```python
from build123d import *

# Parameters (mm, degrees)
CROQUIS1_R                 = 15
SALIENTE_EXTRUIR1_DEPTH    = 22
CROQUIS2_R                 = 10.5
CORTAR_EXTRUIR1_DEPTH      = 16
CORTAR_EXTRUIR2_START      = -1
CORTAR_EXTRUIR2_DEPTH      = 1
CORTAR_EXTRUIR3_START      = -1
CROQUIS5_R                 = 11
CROQUIS5_R_2               = 10.5
CORTAR_EXTRUIR3_DEPTH      = 1
CORTAR_EXTRUIR4_DEPTH      = 31.56141358
CORTAR_EXTRUIR4_DEPTH_BACK = 31.56141358
CROQUIS6_R                 = 1.25


with BuildPart() as part:
    # Croquis1 → Saliente-Extruir1 (new body)
    with BuildSketch(Plane.XY):
        Circle(CROQUIS1_R)
    extrude(amount=SALIENTE_EXTRUIR1_DEPTH)

    # Croquis2 → Cortar-Extruir1 (cut)
    with BuildSketch(Plane.XY.offset(22)):
        Circle(CROQUIS2_R)
    extrude(amount=-CORTAR_EXTRUIR1_DEPTH, mode=Mode.SUBTRACT)

    # Croquis3 → Cortar-Extruir2 (cut)
    with BuildSketch(Plane(origin=(0, 0, 0), x_dir=(-1, 0, 0), z_dir=(0, 0, -1)).offset(CORTAR_EXTRUIR2_START)):
        with BuildLine():
            ThreePointArc((1.25, 10.425329731), (0, 10.5), (-1.25, 10.425329731))
            Line((-1.25, 10.425329731), (-1.25, 9.5))
            Line((-1.25, 9.5), (1.25, 9.5))
            Line((1.25, 9.5), (1.25, 10.425329731))
        make_face()
        with BuildLine():
            Line((-7.602241336, 5.832531755), (-8.40360039, 6.29519662))
            ThreePointArc((-8.40360039, 6.29519662), (-9.09326674, 5.25), (-9.65360039, 4.130133111))
            Line((-9.65360039, 4.130133111), (-8.852241336, 3.667468245))
            Line((-8.852241336, 3.667468245), (-7.602241336, 5.832531755))
        make_face()
        with BuildLine():
            ThreePointArc((9.65360039, 4.130133111), (9.09326674, 5.25), (8.40360039, 6.29519662))
            Line((8.40360039, 6.29519662), (7.602241336, 5.832531755))
            Line((7.602241336, 5.832531755), (8.852241336, 3.667468245))
            Line((8.852241336, 3.667468245), (9.65360039, 4.130133111))
        make_face()
        with BuildLine():
            ThreePointArc((8.40360039, -6.29519662), (9.09326674, -5.25), (9.65360039, -4.130133111))
            Line((9.65360039, -4.130133111), (8.852241336, -3.667468245))
            Line((8.852241336, -3.667468245), (7.602241336, -5.832531755))
            Line((7.602241336, -5.832531755), (8.40360039, -6.29519662))
        make_face()
        with BuildLine():
            Line((-1.25, -9.5), (-1.25, -10.425329731))
            ThreePointArc((-1.25, -10.425329731), (0, -10.5), (1.25, -10.425329731))
            Line((1.25, -10.425329731), (1.25, -9.5))
            Line((1.25, -9.5), (-1.25, -9.5))
        make_face()
        with BuildLine():
            Line((-8.852241336, -3.667468245), (-9.65360039, -4.130133111))
            ThreePointArc((-9.65360039, -4.130133111), (-9.09326674, -5.25), (-8.40360039, -6.29519662))
            Line((-8.40360039, -6.29519662), (-7.602241336, -5.832531755))
            Line((-7.602241336, -5.832531755), (-8.852241336, -3.667468245))
        make_face()
    extrude(amount=CORTAR_EXTRUIR2_DEPTH, mode=Mode.SUBTRACT)

    # Croquis5 → Cortar-Extruir3 (cut)
    with BuildSketch(Plane(origin=(0, 0, 0), x_dir=(-1, 0, 0), z_dir=(0, 0, -1)).offset(CORTAR_EXTRUIR3_START)):
        Circle(CROQUIS5_R)
        with Locations(Location((0, 0, 0), (0, 0, 180))):
            Circle(CROQUIS5_R_2, mode=Mode.SUBTRACT)
    extrude(amount=CORTAR_EXTRUIR3_DEPTH, mode=Mode.SUBTRACT)

    # Croquis6 → Cortar-Extruir4 (cut, two sides: drawn at the far end of the back side and taken through both)
    with BuildSketch(Plane(origin=(0, 0, 0), x_dir=(-1, 0, 0), z_dir=(0, 0, -1)).offset(-CORTAR_EXTRUIR4_DEPTH_BACK)):
        with Locations(Location((0, 0, 0), (0, 0, 180))):
            Circle(CROQUIS6_R)
    extrude(amount=CORTAR_EXTRUIR4_DEPTH + CORTAR_EXTRUIR4_DEPTH_BACK, mode=Mode.SUBTRACT)


solid = part.part
```
Model file for the job. Use its own axes, mm. A direction names the side the tool comes from. Coordinates: 2 decimals unless noted, no trailing zeros. Loops run counter-clockwise (first coordinate to the right, second up) from the corner with the lowest first, then second, coordinate; pieces in that order, holes last. Notation, with made-up numbers: (-16.5, -4.75) - (8.5, -4.75) arc R4 cw to (8.5, 1.25) - close; hole circle Ø4 at (21, 71). An arc over 180 degrees is marked (long way). Write item = value, one per line. Start each with the question number.
Item 1: Pull direction Y, two halves, no side cores. Call faces 1 (the face through (-14.985, 0.66, 10.846)), 2 (the face through (10, 3.2, 14.1)), 3 (the face through (-8, -6.06, 0.51)), 4 (the face through (3.1, 10.2, 22)): +Y half, -Y half, draft (parallel to the pull), parting line (faces both ways), or undercut.
Item 2: Wall check: probe 1 along Y at (x, z) = (0, 0.3); probe 2 along Y at (x, z) = (0, 1.65); probe 3 along Y at (x, z) = (0, 14). Give the ranges that are in metal, low to high. Write a range as [from, to].
Item 3: Drop flat-ended pins along their axis: pin 1 Ø4 at (y, z) = (3, 19.5) entering from -X; pin 2 Ø0.5 at (y, z) = (-10, 0.5) entering from -X; pin 3 Ø2 at (y, z) = (12, 17.5) entering from -X; pin 4 Ø1.5 at (x, y) = (0, 0) entering from -Z. Give the stop position or say it passes through.
Item 4: Saw through at A-A, the plane x = 0. List the corners of the cut face in (y, z), then the cut area to 3 significant figures.
Item 5: 3-axis set-ups, long thin cutter, end or side, ignore diameter. For faces 5 (the face through (-1.25, -0.05, 3.04)), 6 (the face through (-1.25, 10, 0.5)): which of +Z, -Z, +X, -X, +Y, -Y reach the whole face in a straight line?
Item 6: Saw through at D-D, the plane x = -3.5. List the corners of the cut face in (y, z).
Item 7: Saw through at B-B, the plane y = 0. List the corners of the cut face in (x, z).
Item 8: Saw through at C-C, the plane x = 3.25. List the corners of the cut face in (y, z), then the cut area to 3 significant figures.
Answers:
q1.face_1 = parting line
q1.face_2 = undercut
q1.face_3 = undercut
q1.face_4 = draft
q2.probe_1 = [-15, -11], [-9.5, -1.25], [1.25, 9.5], [11, 15]
q2.probe_2 = [-15, -1.25], [1.25, 15]
q2.probe_3 = [-15, -10.5], [10.5, 15]
q3.pin_1 = -14.97
q3.pin_2 = -11.4
q3.pin_3 = -10.2
q3.pin_4 = through
q4.outline = (-15, 0) - (-11, 0) - (-11, 1) - (-9.5, 1) - (-9.5, 0) - (-1.25, 0) - (-1.25, 6) - (-10.5, 6) - (-10.5, 22) - (-15, 22) - close; (1.25, 0) - (9.5, 0) - (9.5, 1) - (11, 1) - (11, 0) - (15, 0) - (15, 22) - (10.5, 22) - (10.5, 6) - (1.25, 6) - close
q4.area = 306 mm2
q5.face_5 = +Z, -Z
q5.face_6 = -Z
q6.outline = (-14.59, 0) - (-10.43, 0) - (-10.43, 1) - (-9.9, 1) - (-9.9, 0) - (9.9, 0) - (9.9, 1) - (10.43, 1) - (10.43, 0) - (14.59, 0) - (14.59, 22) - (9.9, 22) - (9.9, 6) - (-9.9, 6) - (-9.9, 22) - (-14.59, 22) - close
q7.outline = (-15, 0) - (-11, 0) - (-11, 1) - (-10.5, 1) - (-10.5, 0) - (-1.25, 0) - (-1.25, 6) - (-10.5, 6) - (-10.5, 22) - (-15, 22) - close; (1.25, 0) - (10.5, 0) - (10.5, 1) - (11, 1) - (11, 0) - (15, 0) - (15, 22) - (10.5, 22) - (10.5, 6) - (1.25, 6) - close
q8.outline = (-14.64, 0) - (-10.51, 0) - (-10.51, 1) - (-9.98, 1) - (-9.98, 0) - (9.98, 0) - (9.98, 1) - (10.51, 1) - (10.51, 0) - (14.64, 0) - (14.64, 22) - (9.98, 22) - (9.98, 6) - (-9.98, 6) - (-9.98, 22) - (-14.64, 22) - close
q8.area = 324 mm2
